Geometry: final body of the model. Coordinates: model frame, mm. A direction names the side the tool comes from. Round coordinates to 2 decimals unless told otherwise and drop trailing zeros. Loops run counter-clockwise (first coordinate to the right, second up) from the corner with the lowest first, then second, coordinate; pieces in that order, holes last. Notation, with made-up numbers: (44, 78) - (67, 78) arc R13 cw to (67, 83) - close; hole circle Ø1 at (61.5, -15). An arc over 180 degrees is marked (long way). Use CSV: the item, a comma, the result in double quotes.
from build123d import *

# Parameters (mm, degrees)
F0_W          = 20
F0_H          = 376.8444419045
F6_END_RADIUS = 124
F5_R          = 12
F6_REACH      = 357.942125497
F4_R          = 10
F7_DEPTH      = 30
F9_R          = 12
F9_R_2        = 10
F11_R         = 10
F12_DEPTH     = 30
F13_R         = 5
F14_DEPTH     = 10
F15_R         = 5
F16_DEPTH     = 10


with BuildPart() as f1:
    # F0 (on Front) → F1 (revolve)
    with BuildSketch(Plane.XZ):
        with BuildLine():
            Line((-100, 12.7016653793), (-100, 400))
            Line((-100, 400), (-102, 400))
            Line((-102, 400), (-124, 400))
            Line((-124, 400), (-174, 400))
            Line((-174, 400), (-174, 390))
            Line((-174, 390), (-124, 390))
            Line((-124, 390), (-124, 11.1555580955))
            Line((-124, 11.1555580955), (-102, 11.1555580955))
            ThreePointArc((-102, 11.1555580955), (-64.7900629275, 3.2554376606), (-27, -1.0922587136))
            Line((-27, -1.0922587136), (-27, -39.2179855668))
            Line((-27, -39.2179855668), (-75, -39.2179855668))
            Line((-75, -39.2179855668), (-75, -49.2179855668))
            Line((-75, -49.2179855668), (-25, -49.2179855668))
            Line((-25, -49.2179855668), (-25, 0.7820144332))
            ThreePointArc((-25, 0.7820144332), (-62.7835131198, 4.9579383403), (-100, 12.7016653793))
        make_face()
        with Locations((-112, 201.5777790478)):
            Rectangle(F0_W, F0_H, mode=Mode.SUBTRACT)
    revolve(axis=Axis((0, 0, 200), (0, 0, 1)))

    f6_end = (Plane(origin=(0, 0, 200.5777790478), x_dir=(-1, 0, 0), z_dir=(0, 0, -1)) * Cylinder(F6_END_RADIUS, 2048.5579523277, mode=Mode.PRIVATE)).faces().sort_by_distance((124, 0, 200.5777790478))[0]
    # F5 (on offset) → F6 (join, up to the whole of a round face its end follows)
    with BuildSketch(Plane.YZ.offset(-150)):
        with Locations((0, 23)):
            Circle(F5_R)
    f6_long = extrude(amount=F6_REACH, mode=Mode.PRIVATE)
    add(split(f6_long, bisect_by=f6_end, keep=Keep.ALL, mode=Mode.PRIVATE).solids().sort_by_distance((-150, 0, 23))[0])

    # F4 (on offset) → F7 (cut)
    with BuildSketch(Plane.YZ.offset(-150)):
        with Locations((0, 23)):
            Circle(F4_R)
    extrude(amount=F7_DEPTH, mode=Mode.SUBTRACT)

    # F9 (on offset) → F10 (join, up to the next surface of F1)
    with BuildSketch(Plane.YZ.offset(150)):
        with Locations((0, 360)):
            Circle(F9_R)
        with Locations((0, 360)):
            Circle(F9_R_2, mode=Mode.SUBTRACT)
    extrude(until=Until.NEXT, dir=(-1, 0, 0))

    # F11 (on offset) → F12 (cut)
    with BuildSketch(Plane.YZ.offset(150)):
        with Locations((0, 360)):
            Circle(F11_R)
    extrude(amount=-F12_DEPTH, mode=Mode.SUBTRACT)

    # F13 (on face) → F14 (cut, through all)
    with BuildSketch(Plane(origin=(0, 0, -49.2179855668), x_dir=(1, 0, 0), z_dir=(0, 0, -1))):
        with Locations((0, 60)):
            Circle(F13_R)
        with Locations((60, 0)):
            Circle(F13_R)
        with Locations((0, -60)):
            Circle(F13_R)
        with Locations((-60, 0)):
            Circle(F13_R)
    extrude(amount=-F14_DEPTH, mode=Mode.SUBTRACT)

    # F15 (on face) → F16 (cut, through all)
    with BuildSketch(Plane.XY.offset(400)):
        with Locations((0, 160)):
            Circle(F15_R)
        with Locations((-113.1370849898, 113.1370849898)):
            Circle(F15_R)
        with Locations((-160, 0)):
            Circle(F15_R)
        with Locations((-113.1370849898, -113.1370849898)):
            Circle(F15_R)
        with Locations((0, -160)):
            Circle(F15_R)
        with Locations((113.1370849898, -113.1370849898)):
            Circle(F15_R)
        with Locations((160, 0)):
            Circle(F15_R)
        with Locations((113.1370849898, 113.1370849898)):
            Circle(F15_R)
    extrude(amount=-F16_DEPTH, mode=Mode.SUBTRACT)


solid = f1.part
Item 1: Section A-A on z = 23. Return the cut outline in (x, y).
Final values:
outline,"(-150, -12) - (-123.42, -12) arc R124 ccw (long way) to (-123.42, 12) - (-150, 12) - (-150, 10) - (-121.59, 10) arc R122 cw (long way) to (-121.59, -10) - (-150, -10) - close; circle Ø204 at (0, 0); hole circle Ø200 at (0, 0)"
Item 2: Section B-B on x = 132. Return the cut outline in (y, z).
Final values:
outline,"(-113.37, 390) - (113.37, 390) - (113.37, 400) - (-113.37, 400) - close; circle Ø24 at (0, 360); hole circle Ø20 at (0, 360)"
Item 3: Material intervals for line 1 (Z direction, x = 137, y = 0); line 2 (X direction, y = 53, z = 127); line 3 (Y direction, x = 90, z = 289.5), sorted ascending.
Final values:
line 1,"z = 348 to 350, 370 to 372, 390 to 400"
line 2,"x = -112.1 to -109.89, -87.15 to -84.8, 84.8 to 87.15, 109.89 to 112.1"
line 3,"y = -85.3 to -82.37, -48 to -43.59, 43.59 to 48, 82.37 to 85.3"
Item 4: Mould query, pull axis Z, two halves, no side actions, for faces 1 (the flat face through (75, 75, 400)), 2 (the cylindrical face through (155, 0, 395)), 3 (the cylindrical face through (-135, -10, 23)). Classes: released by +Z, released by -Z, zero draft, split by the parting line, or undercut.
Final values:
face 1,"released by +Z"
face 2,"zero draft"
face 3,"undercut"
Item 5: Section C-C on z = 216.5. Return the cut outline in (x, y), plus the area to 3 significant figures.
Final values:
outline,"circle Ø248 at (0, 0); circle Ø204 at (0, 0); hole circle Ø244 at (0, 0); hole circle Ø200 at (0, 0)"
area,"2,810 mm²"
Item 6: Pin query (flat end, axial travel): P1, Ø8, axis at x = 15.5, z = 345, coming from the -Y side; P2, Ø23, axis at y = 0, z = 23, coming from the -X side; P3, Ø16, axis at x = 0, y = 60, coming from the +Z side. Return the tip coordinate at first contact, or that it passes through.
Final values:
P1,"stops at y = -123.47"
P2,"stops at x = -150"
P3,"stops at z = 5.82"
Item 7: Reachability of faces 4 (the flat face through (-150, -5, 32)), 5 (the flat face through (150, -5, 369)), 6 (the cylindrical face through (22.112, 99.574, 204.216)), 7 (the flat face through (47, 91, 11.156)), 8 (the cylindrical face through (-95.38, -30.04, 209.06)) from +Z, -Z, +X, -X, +Y, -Y: full face, straight path, thin tool, end or side. Return the list, or none.
Final values:
face 4,"-Z, -X, +Y, -Y"
face 5,"-Z, +X, +Y, -Y"
face 6,"none"
face 7,"-Z"
face 8,"+Z"
Item 8: Section D-D on x = -81. Return the cut outline in (y, z) (3 decimals), plus the area to 3 significant figures.
Final values:
outline,"(-153.997, 390) - (-93.888, 390) - (-93.888, 11.156) - (-61.992, 11.156) arc R393.755 ccw to (61.992, 11.156) - (93.888, 11.156) - (93.888, 390) - (153.997, 390) - (153.997, 400) - (58.643, 400) - (58.643, 12.702) arc R391.713 cw to (-58.643, 12.702) - (-58.643, 400) - (-153.997, 400) - close; hole (-91.23, 13.156) - (-61.992, 13.156) - (-61.992, 390) - (-91.23, 390) - close; hole (61.992, 13.156) - (91.23, 13.156) - (91.23, 390) - (61.992, 390) - close"
area,"6,820 mm²"
